Read the model definition and answer for the solid it produces. Units are mm, in the model's axes. Give positions to 0.01 mm unless a question says otherwise; leave off trailing zeros. Loops run counter-clockwise (first coordinate to the right, second up) from the corner with the lowest first, then second, coordinate; pieces in that order, holes last. Notation, with made-up numbers: (-1, -8) - (46, -8) arc R18 ccw to (46, 24) - close; hole circle Ø11 at (33, 26.25). An arc over 180 degrees is marked (long way). Write each question's results on one line, items separated by ' | '. Start each with the question number.
Q1. Find the intervals of material crossed by line 1 (X direction, y = 0.1, z = -1.1); line 2 (X direction, y = -0.5, z = -0.6); line 3 (Y direction, x = 13.5, z = 1.85), in increasing order. Write a range as from..to.
Q2. Given pin 1 (2 mm diameter, centred on y = -1.5, z = -0.5, fed in from -X); pin 2 (1.5 mm diameter, centred on y = -1, z = 0.5, fed in from +X), each flat-ended and moving along its own axis, determine where each tip first touches the part or whether it passes through.
Q3. The part is cut by section A-A, the plane z = 0.3. Write down the section's boundary in (x, y).
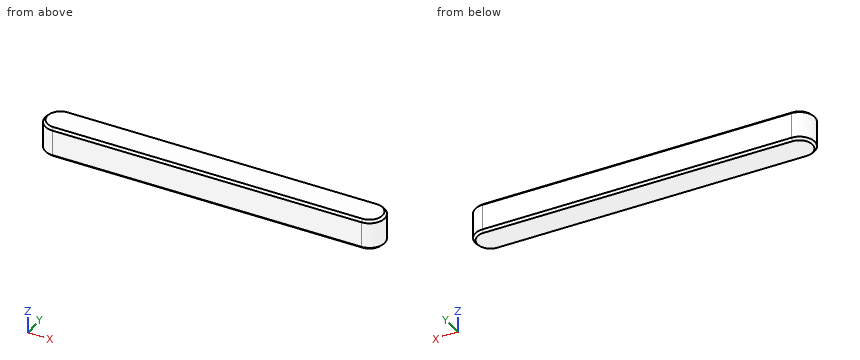
```python
from build123d import *

# Parameters (mm, degrees)
EXTRUDE_1_DEPTH = 2
CHAMFER_1_SIZE  = 0.3


with BuildPart() as part:
    # 草图1 → 凸台-拉伸1 (new, symmetric)
    with BuildSketch(Plane.XY):
        with BuildLine():
            Line((-20, 2), (20, 2))
            ThreePointArc((20, 2), (22, 0), (20, -2))
            Line((20, -2), (-20, -2))
            ThreePointArc((-20, -2), (-22, 0), (-20, 2))
        make_face()
    extrude(amount=EXTRUDE_1_DEPTH, both=True)

    # 倒角1
    chamfer_1_edges = [part.edges().sort_by_distance(p)[0] for p in [
        (22, 0, 2),
        (0, 2, 2),
        (-22, 0, 2),
        (0, 2, -2),
        (22, 0, -2),
        (0, -2, -2),
        (-22, 0, -2),
        (0, -2, 2),
    ]]
    chamfer(chamfer_1_edges, length=CHAMFER_1_SIZE)


solid = part.part
```
Check sheet entries:
1) line 1: x = -22..22 | line 2: x = -21.94..21.94 | line 3: y = -1.85..1.85
2) pin 1: stops at x = -21.94 | pin 2: stops at x = 21.98
3) outline: (-20, -2) - (20, -2) arc R2 ccw to (20, 2) - (-20, 2) arc R2 ccw to start
